from build123d import *

# Parameters (mm, degrees)
BOSS_EXTRUDE1_DEPTH = 0.912
SKETCH1_3_W         = 16.55774554
SKETCH1_3_H         = 15.901271047
BOSS_EXTRUDE2_DEPTH = 5.08
BOSS_EXTRUDE3_DEPTH = 5.08


with BuildPart() as part:
    # Sketch1 → Boss-Extrude1 (new body)
    with BuildSketch(Plane(origin=(0, 0, 0), x_dir=(0, 0, -1), z_dir=(1, 0, 0))):
        Polygon((0, 0), (5.014983062, 0), (5.014983062, 20.218431916), (10.514983062, 20.218431916), (10.514983062, 0), (30.0377124, 0), (30.0377124, 9.933664863), (13.47996686, 9.933664863), (13.47996686, 25.83493591), (0, 25.83493591), align=None)
    extrude(amount=-BOSS_EXTRUDE1_DEPTH)

    # Sketch1_3 → Boss-Extrude2 (add)
    with BuildSketch(Plane(origin=(0, 0, 0), x_dir=(0, 0, -1), z_dir=(1, 0, 0))):
        with Locations((21.75883963, 17.884300387)):
            Rectangle(SKETCH1_3_W, SKETCH1_3_H)
        Polygon((0, 0), (5.014983062, 0), (5.014983062, 20.218431916), (10.514983062, 20.218431916), (10.514983062, 0), (30.0377124, 0), (30.0377124, 9.933664863), (13.47996686, 9.933664863), (13.47996686, 25.83493591), (0, 25.83493591), align=None)
    extrude(amount=BOSS_EXTRUDE2_DEPTH)

    # Sketch2 → Boss-Extrude3 (add)
    with BuildSketch(Plane.ZY.offset(0.912)):
        Polygon((-30.0377124, 25.83493591), (0, 25.83493591), (0, 0), (-5.014983062, 0), (-5.014983062, 20.218431916), (-10.514983062, 20.218431916), (-10.514983062, 0), (-30.0377124, 0), align=None)
    extrude(amount=BOSS_EXTRUDE3_DEPTH)


solid = part.part
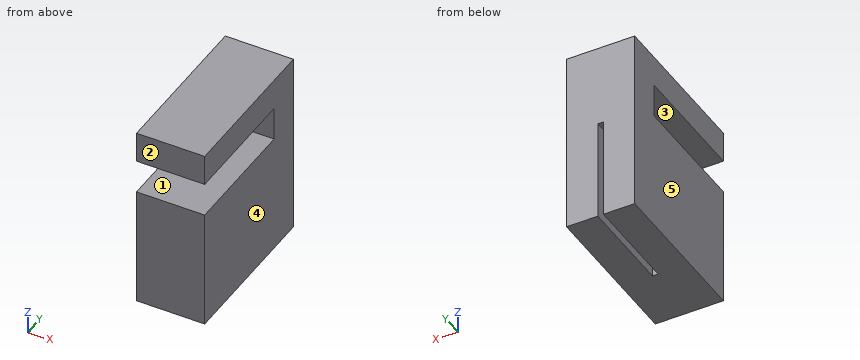
CAD build for the part. Positions are in the model's coordinates, mm. Face numbers are marked on the shaded views. A direction names the side the tool comes from. Round coordinates to 2 decimals unless told otherwise and drop trailing zeros. Write each loop counter-clockwise with the first axis right and the second up, starting at its lowest first coordinate (ties: lowest second). Pieces come first, ordered by that corner, then holes.
(1) Slice it at D-D, the plane y = 3.5. Write the cut outline in (x, z), and give its area (3 significant figures).
(2) Probe line 1 along Z through (x, y) = (-0.75, 13); line 2 along Z through (x, y) = (4, 4.5); line 3 along X through (y, z) = (19.25, -20). List the from-to ranges inside material, lowest first.
(3) Slice it at B-B, the plane z = -16. Write the cut outline in (x, y), and give its area (3 significant figures).
(4) 3-axis set-ups, long thin cutter, end or side, ignore diameter. For the marked faces 1 and 2: which of +Z, -Z, +X, -X, +Y, -Y reach the whole face in a straight line?
(5) Drop flat-ended pins along their axis: P1, Ø1, axis at x = -3.5, z = -13.5, coming from the -Y side; P2, Ø3, axis at x = 0, z = -8.5, coming from the -Y side; P3, Ø0.7, axis at x = -0.5, y = 16, coming from the -Z side. Give the stop position or say it passes through.
(6) Mould opens along X. For the marked faces 3, 4 and 5 say: pulls with the +X half, pulls with the -X half, needs draft (parallel to the pull), parting line crosses it, or undercut.
(7) Slice it at A-A, the plane y = 18.5. Write the cut outline in (x, z).
(8) Slice it at C-C, the plane y = 21.75. Write the cut outline in (x, z).
From the geometry:
1. outline: (-5.99, -30.04) - (5.08, -30.04) - (5.08, -10.51) - (-5.99, -10.51) - close; (-5.99, -5.01) - (5.08, -5.01) - (5.08, 0) - (-5.99, 0) - close
1. area: 272 mm2
2. line 1: z = -13.48 to -10.51, -5.01 to 0
2. line 2: z = -30.04 to -10.51, -5.01 to 0
2. line 3: x = -5.99 to -0.91, 0 to 5.08
3. outline: (-5.99, 0) - (5.08, 0) - (5.08, 25.83) - (0, 25.83) - (0, 9.93) - (-0.91, 9.93) - (-0.91, 25.83) - (-5.99, 25.83) - close
3. area: 272 mm2
4. face 1: +X, -X, -Y
4. face 2: +Z, -Z, +X, -X, -Y
5. P1: stops at y = 0
5. P2: stops at y = 20.22
5. P3: stops at z = -13.48
6. face 3: needs draft
6. face 4: pulls with the +X half
6. face 5: pulls with the -X half
7. outline: (-5.99, -30.04) - (-0.91, -30.04) - (-0.91, -13.48) - (0, -13.48) - (0, -30.04) - (5.08, -30.04) - (5.08, -10.51) - (-5.99, -10.51) - close; (-5.99, -5.01) - (5.08, -5.01) - (5.08, 0) - (-5.99, 0) - close
8. outline: (-5.99, -30.04) - (-0.91, -30.04) - (-0.91, -13.48) - (0, -13.48) - (0, -30.04) - (5.08, -30.04) - (5.08, 0) - (-5.99, 0) - close
